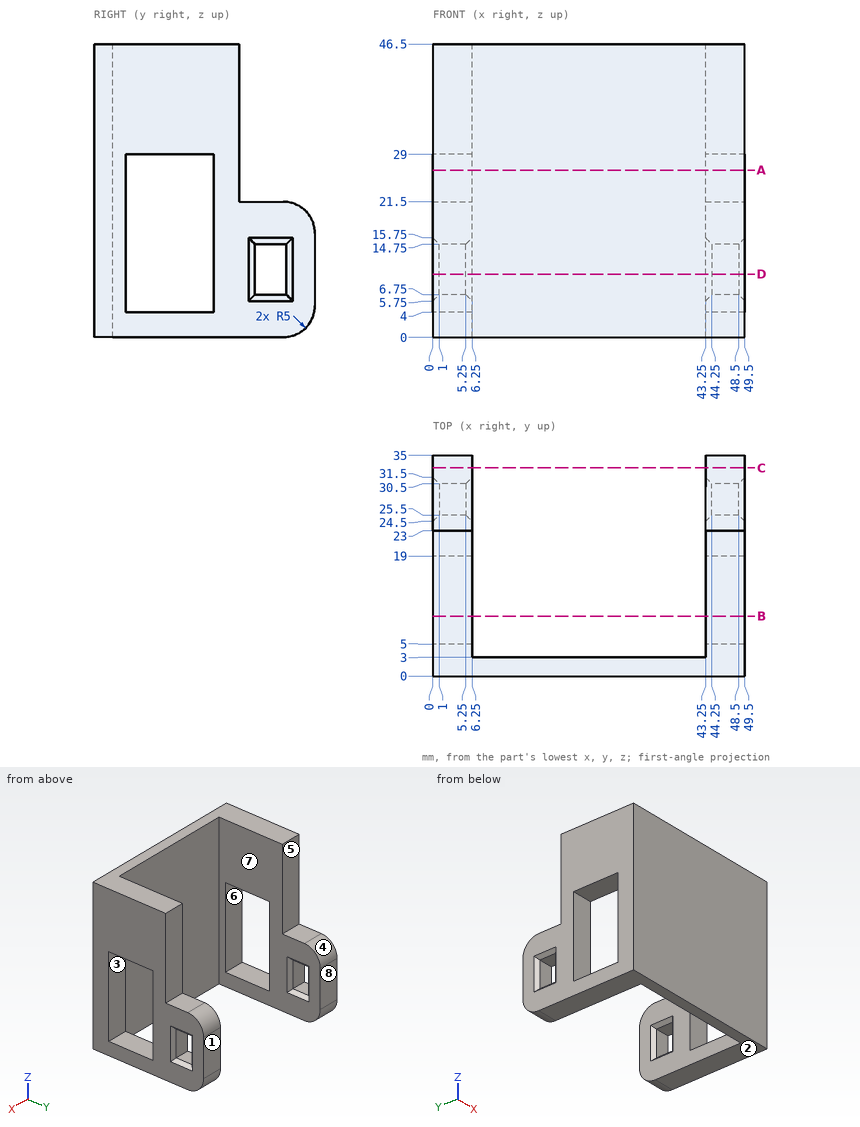
Verification items for this drawing (mm, ordinates from the low corner). A direction names the side the tool comes from. Coordinates: 2 decimals unless noted, no trailing zeros. Order: outer loops, then holes, each group sorted by start corner. A loop starts at its lowest first (then second) coordinate and runs counter-clockwise, first axis right, second up. Notation, with made-up numbers: (24, 88) - (81, 88) arc R32 cw to (81, 123) - close; hole circle Ø3 at (-34.5, -12.5). An arc over 180 degrees is marked (long way). Answer in a Markdown table with one row per item. Add a question column.
1. Section check D-D (z = 10). Give the number of separate pieces and of enclosed holes in the cut face, plus the area to 3 significant figures.
2. Section check C-C (y = 33). Enter the section's corners in (x, z), plus the area to 3 significant figures.
3. Section check B-B (y = 9.5). Enter the section's corners in (x, z).
4. Draft check along Z on the marked faces 1, 2, 3 and 4. Enter one of: +Z half, -Z half, draft (parallel to the pull), parting line (faces both ways), or undercut.
5. Material ranges on L1, parallel to Z at x = 45, y = 13.5; L2, parallel to X at y = 21, z = 45; L3, parallel to Y at x = 34, z = 42.5, recorded low to high. Write a range as [from, to].
6. Access from +Z, -Z, +X, -X, +Y, -Y to the whole of each face (thin tool, end or side, straight path). Record for the marked faces 5, 6, 7 and 8.
7. Section check A-A (z = 26.5). Enter the section's corners in (x, y).
8. Gauge pin test, flat ends, axial feed: pin 1 Ø1.5 at (x, z) = (34.5, 38.5) entering from +Y; pin 2 Ø5 at (x, y) = (4.5, 26.5) entering from +Z; pin 3 Ø5 at (x, z) = (3, 39.5) entering from +Y. Record the tip position at first contact, or that the pin passes through.
Data:
| question | item | result |
|---|---|---|
| 1 | separate pieces | 5 |
| 1 | enclosed holes | 0 |
| 1 | area | 307 mm² |
| 2 | outline | (0, 1) - (6.25, 1) - (6.25, 20.5) - (0, 20.5) - close; (43.25, 1) - (49.5, 1) - (49.5, 20.5) - (43.25, 20.5) - close |
| 2 | area | 244 mm² |
| 3 | outline | (0, 0) - (6.25, 0) - (6.25, 4) - (0, 4) - close; (0, 29) - (6.25, 29) - (6.25, 46.5) - (0, 46.5) - close; (43.25, 0) - (49.5, 0) - (49.5, 4) - (43.25, 4) - close; (43.25, 29) - (49.5, 29) - (49.5, 46.5) - (43.25, 46.5) - close |
| 4 | face 1 | draft |
| 4 | face 2 | -Z half |
| 4 | face 3 | undercut |
| 4 | face 4 | +Z half |
| 5 | L1 | z = [0, 4], [29, 46.5] |
| 5 | L2 | x = [0, 6.25], [43.25, 49.5] |
| 5 | L3 | y = [0, 3] |
| 6 | face 5 | +Z, +X, -X, +Y |
| 6 | face 6 | +X, -X |
| 6 | face 7 | +Z, -Z, +Y |
| 6 | face 8 | +Z, -Z, +X, -X, +Y |
| 7 | outline | (0, 0) - (49.5, 0) - (49.5, 5) - (43.25, 5) - (43.25, 3) - (6.25, 3) - (6.25, 5) - (0, 5) - close; (0, 19) - (6.25, 19) - (6.25, 23) - (0, 23) - close; (43.25, 19) - (49.5, 19) - (49.5, 23) - (43.25, 23) - close |
| 8 | pin 1 | stops at y = 3 |
| 8 | pin 2 | stops at z = 21.5 |
| 8 | pin 3 | stops at y = 23 |
